Autodesk Inventor part; units mm, degrees
ref_plane "Work Plane1" through (0, 0, 40) normal (1, 0, 0) x (0, 0, -1)
ref_plane "Work Plane2" through (0, 75, 0) normal (0, -1, 0) x (1, 0, 0)
ref_plane "Work Plane3" through (40, 0, 0) normal (0, 0, -1) x (-1, 0, 0)
sketch "Sketch1" plane through (0, 0, 0) normal (0, 1, 0) x (-1, 0, 0)
  line L0 (40, 40) -> (-40, 40)
  line L1 (-40, 40) -> (-40, -40)
  line L2 (-40, -40) -> (40, -40)
  line L3 (40, -40) -> (40, 40)
  line L4 (40, 40) -> (-40, -40) construction
  line L5 (-40, 40) -> (40, -40) construction
  point P0 (0, 0)
  dimension "d0" = 80
  dimension "d1" = 80
extrude "Extrusion1" add sketch "Sketch1" along normal blind 10
sketch "Sketch2" plane through (0, 10, 0) normal (0, 1, 0) x (1, 0, 0)
  circle A0 centre (30, 30) radius 3.1
  circle A1 centre (30, -30) radius 3.1
  circle A2 centre (-30, -30) radius 3.1
  circle A3 centre (-30, 30) radius 3.1
  point P0 (0, 0)
  dimension "d4" = 6.2
  dimension "d5" = 6.2
  dimension "d6" = 6.2
  dimension "d7" = 6.2
  dimension "d8" = 30
  dimension "d9" = 30
  dimension "d10" = 30
  dimension "d11" = 30
  dimension "d12" = 30
  dimension "d13" = 30
  dimension "d14" = 30
  dimension "d15" = 30
extrude "Extrusion2" cut sketch "Sketch2" against normal blind 10
sketch "Sketch3" plane through (0, 10, 0) normal (0, 1, 0) x (1, 0, 0)
  line L0 (40, 10) -> (-40, 10)
  line L1 (-40, 10) -> (-40, 20)
  line L2 (-40, 20) -> (40, 20)
  line L3 (40, 20) -> (40, 10)
  line L4 (40, 10) -> (-40, 20) construction
  line L5 (-40, 10) -> (40, 20) construction
  line L6 (40, -20) -> (-40, -20)
  line L7 (-40, -20) -> (-40, -10)
  line L8 (-40, -10) -> (40, -10)
  line L9 (40, -10) -> (40, -20)
  line L10 (40, -20) -> (-40, -10) construction
  line L11 (-40, -20) -> (40, -10) construction
  line L12 (-40, 40) -> (-40, -40)
  line L13 (40, -40) -> (40, 40)
  line L14 (40, 40) -> (-40, 40)
  line L15 (-40, -40) -> (40, -40)
  point P0 (0, 0)
  point P1 (0, 15)
  point P2 (0, -15)
  dimension "d19" = 10
  dimension "d20" = 10
  dimension "d21" = 20
  dimension "d22" = 20
extrude "Extrusion3" add sketch "Sketch3" along normal blind 130 contours L0 L1 L2 L3 | L9 L6 L7 L8
sketch "Sketch4" plane through (0, 10, 0) normal (0, 1, 0) x (1, 0, 0)
  line L0 (20, -10) -> (-20, -10)
  line L1 (-20, -10) -> (-20, 10)
  line L2 (-20, 10) -> (20, 10)
  line L3 (20, 10) -> (20, -10)
  line L4 (20, -10) -> (-20, 10) construction
  line L5 (-20, -10) -> (20, 10) construction
  line L6 (-40, 10) -> (40, 10)
  point P0 (0, 0)
  dimension "d25" = 40
extrude "Extrusion4" cut sketch "Sketch4" against normal blind 10
sketch "Sketch5" plane through (0, 140, 0) normal (0, 1, 0) x (1, 0, 0)
  line L0 (50, -60) -> (-50, -60)
  line L1 (-50, -60) -> (-50, 60)
  line L2 (-50, 60) -> (50, 60)
  line L3 (50, 60) -> (50, -60)
  line L4 (50, -60) -> (-50, 60) construction
  line L5 (-50, -60) -> (50, 60) construction
  point P0 (0, 0)
  dimension "d28" = 100
  dimension "d29" = 120
extrude "Extrusion5" add sketch "Sketch5" along normal blind 10
sketch "Sketch6" plane through (0, 150, 0) normal (0, 1, 0) x (1, 0, 0)
  circle A0 centre (-40, 50) radius 3.1
  circle A1 centre (40, 50) radius 3.1
  circle A2 centre (40, -50) radius 3.1
  circle A3 centre (-40, -50) radius 3.1
  point P0 (0, 0)
  dimension "d32" = 6.2
  dimension "d33" = 6.2
  dimension "d34" = 6.2
  dimension "d35" = 6.2
  dimension "d36" = 50
  dimension "d37" = 50
  dimension "d38" = 50
  dimension "d39" = 50
  dimension "d40" = 40
  dimension "d41" = 40
  dimension "d42" = 40
  dimension "d43" = 40
extrude "Extrusion6" cut sketch "Sketch6" against normal blind 10
ref_plane "Work Plane1" through (0, 0, 40) normal (1, 0, 0) x (0, 0, -1)
sketch "Sketch7" plane through (0, 0, 40) normal (1, 0, 0) x (0, 0, -1)
  line L0 (80, 10) -> (60, 10)
  line L1 (60, 10) -> (60, 30)
  line L2 (60, 10) -> (80, 10)
  line L3 (60, 10) -> (60, 140)
  line L4 (60, 30) -> (80, 10)
  point P0 (40, 0)
  dimension "d47" = 20
  dimension "d48" = 20
extrude "Extrusion7" add sketch "Sketch7" along normal mid plane 10
ref_plane "Work Plane2" through (0, 75, 0) normal (0, -1, 0) x (1, 0, 0)
mirror "Mirror1" about plane through (0, 75, 0) normal (0, -1, 0) of "Extrusion7"
ref_plane "Work Plane3" through (40, 0, 0) normal (0, 0, -1) x (-1, 0, 0)
mirror "Mirror2" about plane through (40, 0, 0) normal (0, 0, -1) of "Extrusion7", "Mirror1"
properties part number "lidar" material "ABS Plastic"
Model file for the job. Use its own axes, mm. A direction names the side the tool comes from. Give positions to 0.01 mm unless a question says otherwise; leave off trailing zeros. Loops run counter-clockwise (first coordinate to the right, second up) from the corner with the lowest first, then second, coordinate; pieces in that order, holes last. Notation, with made-up numbers: (-7.75, 61) -> (50.25, 61) arc R20 cw to (50.25, 79) -> close; hole circle Ø2 at (-11, 41). An arc over 180 degrees is marked (long way). Write each question's results on one line, items separated by ' | '.
(1) Cut at A-A on x = -30. List the corners of the cut face in (y, z).
Geometry results:
outline: (0, -40) -> (10, -40) -> (10, -33.1) -> (0, -33.1) -> close; (0, -26.9) -> (10, -26.9) -> (10, -20) -> (140, -20) -> (140, -60) -> (150, -60) -> (150, 60) -> (140, 60) -> (140, 20) -> (10, 20) -> (10, 26.9) -> (0, 26.9) -> close; (0, 33.1) -> (10, 33.1) -> (10, 40) -> (0, 40) -> close; hole (10, -10) -> (140, -10) -> (140, 10) -> (10, 10) -> close
(2) Cut at C-C on y = 14.5. List the corners of the cut face in (x, z), and give its area (3 significant figures).
Geometry results:
outline: (-40, -20) -> (-5, -20) -> (-5, -35.5) -> (5, -35.5) -> (5, -20) -> (40, -20) -> (40, -10) -> (-40, -10) -> close; (-40, 10) -> (40, 10) -> (40, 20) -> (5, 20) -> (5, 35.5) -> (-5, 35.5) -> (-5, 20) -> (-40, 20) -> close | area: 1,910 mm²
(3) Tool access for faces 1 (the flat face through (1, 5, -40)), 2 (the flat face through (-5, 134, -26)), 3 (the flat face through (0, 130, -30)): list every direction of +Z, -Z, +X, -X, +Y, -Y with a clear straight run to the whole face (end or side of a thin tool).
Geometry results:
face 1: -Z, +X, -X, -Y | face 2: -Z, -X | face 3: -Z, +X, -X
(4) Cut at B-B on z = -50. List the corners of the cut face in (x, y).
Geometry results:
outline: (-50, 140) -> (-43.1, 140) -> (-43.1, 150) -> (-50, 150) -> close; (-36.9, 140) -> (36.9, 140) -> (36.9, 150) -> (-36.9, 150) -> close; (43.1, 140) -> (50, 140) -> (50, 150) -> (43.1, 150) -> close
(5) Flat gauge pins, fed straight in: pin 1 Ø3.5 at (x, z) = (30, -30) entering from -Y; pin 2 Ø8 at (x, y) = (-2.5, 68.5) entering from -Z; pin 3 Ø24 at (x, y) = (-14, 98.5) entering from +Z. Where does each tip first touch, or does it go through?
Geometry results:
pin 1: stops at y = 140 | pin 2: stops at z = -20 | pin 3: stops at z = 20
(6) Probe line 1 along Z through (x, y) = (-30, 2); line 2 along Z through (x, y) = (40, 145.75). List the from-to ranges inside material, lowest first.
Geometry results:
line 1: z = -40 to -33.1, -26.9 to 26.9, 33.1 to 40 | line 2: z = -60 to -53.1, -46.9 to 46.9, 53.1 to 60
(7) Cut at D-D on z = -36. List the corners of the cut face in (x, y).
Geometry results:
outline: (-50, 140) -> (-5, 140) -> (-5, 136) -> (5, 136) -> (5, 140) -> (50, 140) -> (50, 150) -> (-50, 150) -> close; (-40, 0) -> (40, 0) -> (40, 10) -> (5, 10) -> (5, 14) -> (-5, 14) -> (-5, 10) -> (-40, 10) -> close
(8) Pull direction X, two halves, no side cores. Call faces 4 (the cylindrical face through (-40.404, 145.07, -53.074)), 5 (the flat face through (5, 16, 26)), 6 (the flat face through (-1, 150, -1)): released by +X, released by -X, zero draft, split by the parting line, or undercut.
Geometry results:
face 4: undercut | face 5: released by +X | face 6: zero draft
